Verification items for the finished model (mm, model axes). A direction names the side the tool comes from. Coordinates: 2 decimals unless noted, no trailing zeros. Order: outer loops, then holes, each group sorted by start corner. A loop starts at its lowest first (then second) coordinate and runs counter-clockwise, first axis right, second up.
Q1. Cross-section at B-B, the plane x = 0. Record the boundary of the cut face in (y, z) (1 decimal), and give its area (3 significant figures).
Q2. Set-up check for faces 1 (the cylindrical face through (-7.93, 0.35, 1.55)), 2 (the flat face through (-9.047, -4.247, 4.15)): record each of +Z, -Z, +X, -X, +Y, -Y from which the full face is reachable in a straight line by a thin tool's end or side.
Q3. Draft check along X on faces 3 (the flat face through (-14.288, 0, 4)), 4 (the cylindrical face through (-12.464, 0.059, 4.15)), 5 (the cylindrical face through (9.76, 0.06, 4.15)), 6 (the flat face through (9.047, 4.247, 4.15)). Enter one of: pulls with the +X half, pulls with the -X half, needs draft (parallel to the pull), parting line crosses it, or undercut.
Q4. Depth check by flat-ended pin: P1, Ø1, axis at y = -0.5, z = 1.5, coming from the +X side; P2, Ø1, axis at y = -3.5, z = 1.5, coming from the +X side; P3, Ø3.5, axis at x = -11.11, y = 0, coming from the -Z side; P4, Ø2.5, axis at x = 11.11, y = 0, coming from the -Z side. Enter the tip coordinate at first touch or a pass-through.
Q5. Cross-section at C-C, the plane z = 3.9. Record the boundary of the cut face in (x, y) (1 decimal), and give its area (3 significant figures).
Q6. Thickness scan on line 1 (Y direction, x = 0, z = 2.35); line 2 (X direction, y = 1, z = 4.2); line 3 (Z direction, x = -8.5, y = 2) (3 decimals). Record the ranges inside material, lowest first.
Q7. Cross-section at A-A, the plane y = 0. Record the boundary of the cut face in (x, z) (1 decimal), and give its area (3 significant figures).
Q8. Cross-section at D-D, the plane z = 0.9. Record the boundary of the cut face in (x, y) (1 decimal), and give its area (3 significant figures).
from build123d import *

# Parameters (mm, degrees)
F0_R     = 7.9375
F0_R_2   = 3.96875
F1_DEPTH = 5.715
F2_R     = 1.35255
F3_DEPTH = 3.175


with BuildPart() as f1:
    # F0 (on Top) → F1 (new body)
    with BuildSketch(Plane.XY):
        Circle(F0_R)
        Circle(F0_R_2, mode=Mode.SUBTRACT)
    extrude(amount=F1_DEPTH)

    # F2 (on face) → F3 (join)
    with BuildSketch(Plane.XY.offset(5.715)):
        with BuildLine():
            Line((-3.65679, 7.044983), (-14.2875, 1.526975))
            Line((-14.2875, 1.526975), (-14.2875, -1.526975))
            Line((-14.2875, -1.526975), (-3.65679, -7.044983))
            ThreePointArc((-3.65679, -7.044983), (-7.9375, 0), (-3.65679, 7.044983))
        make_face()
        with Locations((-11.1125, 0)):
            Circle(F2_R, mode=Mode.SUBTRACT)
        with BuildLine():
            Line((14.2875, 1.526975), (3.65679, 7.044983))
            ThreePointArc((3.65679, 7.044983), (6.783424, 4.121779), (7.9375, 0))
            ThreePointArc((7.9375, 0), (6.783424, -4.121779), (3.65679, -7.044983))
            Line((3.65679, -7.044983), (14.2875, -1.526975))
            Line((14.2875, -1.526975), (14.2875, 1.526975))
        make_face()
        with Locations((11.1125, 0)):
            Circle(F2_R, mode=Mode.SUBTRACT)
    extrude(amount=-F3_DEPTH)


solid = f1.part
Check values:
1. outline: (-7.9, 0) - (-4, 0) - (-4, 5.7) - (-7.9, 5.7) - close; (4, 0) - (7.9, 0) - (7.9, 5.7) - (4, 5.7) - close
1. area: 45.4 mm2
2. face 1: -Z
2. face 2: +Z, -Z, -X, -Y
3. face 3: pulls with the -X half
3. face 4: undercut
3. face 5: undercut
3. face 6: pulls with the +X half
4. P1: stops at x = 7.94
4. P2: stops at x = 7.35
4. P3: stops at z = 2.54
4. P4: passes through
5. outline: (-14.3, -1.5) - (-3.7, -7) arc R7.9 ccw to (3.7, -7) - (14.3, -1.5) - (14.3, 1.5) - (3.7, 7) arc R7.9 ccw to (-3.7, 7) - (-14.3, 1.5) - close; hole circle Ø2.7 at (-11.1, 0); hole circle Ø7.9 at (0, 0); hole circle Ø2.7 at (11.1, 0)
5. area: 233 mm2
6. line 1: y = -7.94 to -3.97, 3.97 to 7.94
6. line 2: x = -14.29 to -12.02, -10.2 to -3.84, 3.84 to 10.2, 12.02 to 14.29
6. line 3: z = 2.54 to 5.715
7. outline: (-14.3, 2.5) - (-12.5, 2.5) - (-12.5, 5.7) - (-14.3, 5.7) - close; (-9.8, 2.5) - (-7.9, 2.5) - (-7.9, 0) - (-4, 0) - (-4, 5.7) - (-9.8, 5.7) - close; (4, 0) - (7.9, 0) - (7.9, 2.5) - (9.8, 2.5) - (9.8, 5.7) - (4, 5.7) - close; (12.5, 2.5) - (14.3, 2.5) - (14.3, 5.7) - (12.5, 5.7) - close
7. area: 68.5 mm2
8. outline: circle Ø15.9 at (0, 0); hole circle Ø7.9 at (0, 0)
8. area: 148 mm2
